The figure shows three views and two pictorial views of one solid part (mm, origin at its lowest corner). Answer the questions. Coordinates: 2 decimals unless noted, no trailing zeros. Loops run counter-clockwise (first coordinate to the right, second up) from the corner with the lowest first, then second, coordinate; pieces in that order, holes last. Notation, with made-up numbers: (9, 19.5) - (31, 19.5) arc R29 ccw to (31, 58.5) - close; hole circle Ø9 at (13, -24.75). An arc over 180 degrees is marked (long way). One line per question, with ' | ' between items.
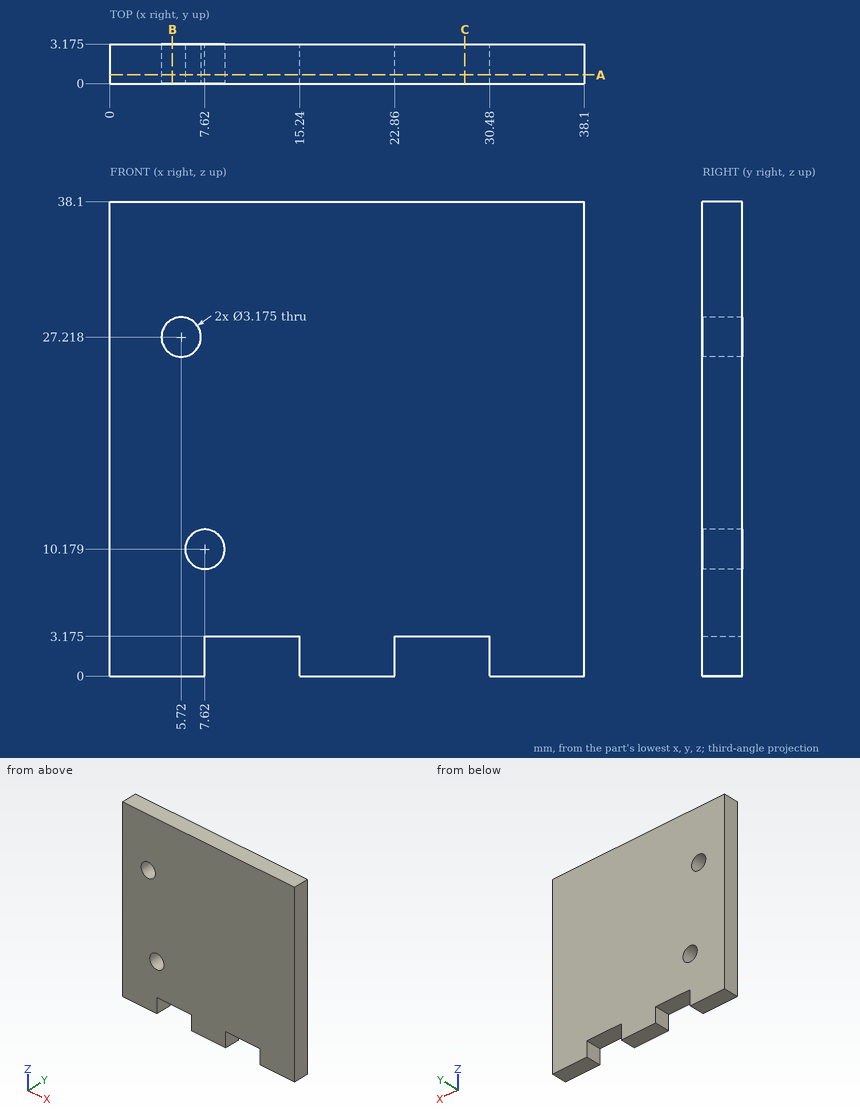
Item 1: Each of these flat-tipped pins is pushed along its axis until it touches: pin 1 Ø1.6 at (x, y) = (25.5, 2) entering from -Z (3 decimals); pin 2 Ø4 at (x, z) = (16.5, 16.5) entering from -Y; pin 3 Ø3 at (x, z) = (7.62, 10.18) entering from +Y. Where does it stop, or does it pass through?
Taken from the geometry:
pin 1: stops at z = 3.175 | pin 2: stops at y = 0 | pin 3: passes through
Item 2: Find section B-B, the plane x = 5. Write down the section's boundary in (y, z) (1 decimal), plus the area to 3 significant figures.
Taken from the geometry:
outline: (0, 0) - (3.2, 0) - (3.2, 25.8) - (0, 25.8) - close; (0, 28.6) - (3.2, 28.6) - (3.2, 38.1) - (0, 38.1) - close | area: 112 mm2
Item 3: Find section A-A, the plane y = 0.7. Write down the section's boundary in (x, z) (1 decimal), plus the area to 3 significant figures.
Taken from the geometry:
outline: (0, 0) - (7.6, 0) - (7.6, 3.2) - (15.2, 3.2) - (15.2, 0) - (22.9, 0) - (22.9, 3.2) - (30.5, 3.2) - (30.5, 0) - (38.1, 0) - (38.1, 38.1) - (0, 38.1) - close; hole circle Ø3.2 at (5.7, 27.2); hole circle Ø3.2 at (7.6, 10.2) | area: 1,390 mm2
Item 4: Find the intervals of material crossed by line 1 (Z direction, x = 23.5, y = 2.45) (1 decimal); line 2 (X direction, y = 2.35, z = 26) (1 decimal); line 3 (X direction, y = 1.45, z = 27), in increasing order. Write a range as [from, to].
Taken from the geometry:
line 1: z = [3.2, 38.1] | line 2: x = [0, 4.7], [6.7, 38.1] | line 3: x = [0, 4.15], [7.29, 38.1]
Item 5: Find section C-C, the plane x = 28.5. Write down the section's boundary in (y, z) (1 decimal), plus the area to 3 significant figures.
Taken from the geometry:
outline: (0, 3.2) - (3.2, 3.2) - (3.2, 38.1) - (0, 38.1) - close | area: 111 mm2
